from build123d import *

# Parameters (mm, degrees)
SKETCH1_W           = 10
SKETCH1_H           = 6
BOSS_EXTRUDE1_DEPTH = 65
SKETCH2_R           = 1.6
CUT_EXTRUDE1_DEPTH  = 67.037867924
FILLET1_R           = 3


with BuildPart() as part:
    # Sketch1 → Boss-Extrude1 (new body)
    with BuildSketch(Plane.XY):
        with Locations((5, -3)):
            Rectangle(SKETCH1_W, SKETCH1_H)
    extrude(amount=BOSS_EXTRUDE1_DEPTH)

    # Sketch2 → Cut-Extrude1 (cut, through all)
    with BuildSketch(Plane(origin=(0, 0, 0), x_dir=(1, 0, 0), z_dir=(0, 1, 0))):
        with Locations(Location((5, -5, 0), (0, 0, 270))):
            Circle(SKETCH2_R)
        with Locations(Location((5, -60, 0), (0, 0, 270))):
            Circle(SKETCH2_R)
    extrude(amount=-CUT_EXTRUDE1_DEPTH, mode=Mode.SUBTRACT)

    # Fillet1
    fillet1_edges = [part.edges().sort_by_distance(p)[0] for p in [
        (10, -3, 65),
        (0, -3, 65),
        (10, -3, 0),
        (0, -3, 0),
    ]]
    fillet(fillet1_edges, radius=FILLET1_R)


solid = part.part
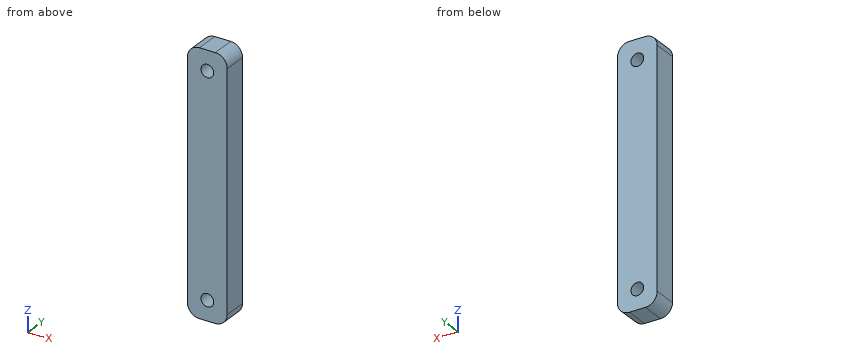
The model under review builds one solid part; all positions refer to its coordinate system, in mm. Coordinates: 2 decimals unless noted, no trailing zeros. Order: outer loops, then holes, each group sorted by start corner. A loop starts at its lowest first (then second) coordinate and runs counter-clockwise, first axis right, second up. Notation, with made-up numbers: (29.5, 65) -> (72.5, 65) arc R29 ccw to (72.5, 96) -> close; hole circle Ø11 at (55, 44.25). An arc over 180 degrees is marked (long way). Answer in a Markdown table with one row per item.
(1) Consider section A-A (x = 5). Write out the cut boundary in (y, z).
Answers:
| item | result |
|---|---|
| outline | (-6, 0) -> (0, 0) -> (0, 3.4) -> (-6, 3.4) -> close; (-6, 6.6) -> (0, 6.6) -> (0, 58.4) -> (-6, 58.4) -> close; (-6, 61.6) -> (0, 61.6) -> (0, 65) -> (-6, 65) -> close |
(2) Wall thickness on line 1 along X through (y, z) = (-4.2, 60); line 2 along Z through (x, y) = (4, -3); line 3 along X through (y, z) = (-1.85, 4): over which ranges is each line inside the solid? List them lowest first.
Answers:
| item | result |
|---|---|
| line 1 | 0 to 3.4, 6.6 to 10 |
| line 2 | 0 to 3.75, 6.25 to 58.75, 61.25 to 65 |
| line 3 | 0 to 3.75, 6.25 to 10 |
(3) Consider section C-C (y = -1.65). Write out the cut boundary in (x, z), plus the area to 3 significant figures.
Answers:
| item | result |
|---|---|
| outline | (0, 3) arc R3 ccw to (3, 0) -> (7, 0) arc R3 ccw to (10, 3) -> (10, 62) arc R3 ccw to (7, 65) -> (3, 65) arc R3 ccw to (0, 62) -> close; hole circle Ø3.2 at (5, 5); hole circle Ø3.2 at (5, 60) |
| area | 626 mm² |
(4) Insertion check: pin 1 (1 mm diameter, centred on x = 8.5, y = -4, fed in from -Z). The pin has a flat end and moves straight along its axis. Give the tip position at first contact, or say it passes through.
Answers:
| item | result |
|---|---|
| pin 1 | z = 0.17 |
(5) Consider section B-B (z = 60). Write out the cut boundary in (x, y).
Answers:
| item | result |
|---|---|
| outline | (0, -6) -> (3.4, -6) -> (3.4, 0) -> (0, 0) -> close; (6.6, -6) -> (10, -6) -> (10, 0) -> (6.6, 0) -> close |
